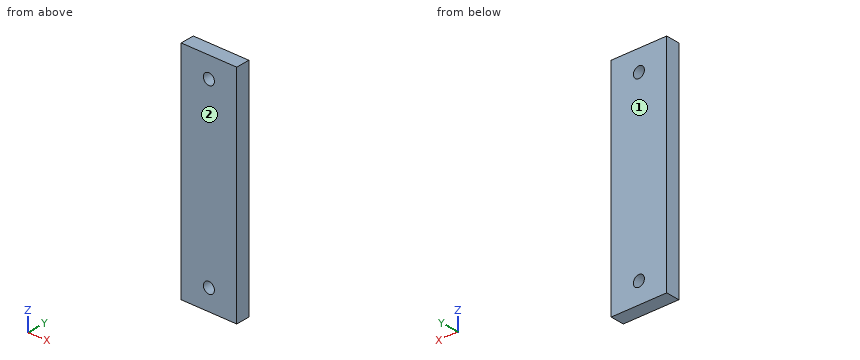
```python
from build123d import *

# Parameters (mm, degrees)
F0_W     = 50.8
F0_H     = 203.2
F1_DEPTH = 12.7
F2_D     = 10.0838
F2_DEPTH = 12.7
F2_TIP   = 3.0294791551


with BuildPart() as f1:
    # F0 (on Front) → F1 (new body)
    with BuildSketch(Plane.XZ):
        Rectangle(F0_W, F0_H)
    extrude(amount=F1_DEPTH)

    # F2
    with Locations(Plane(origin=(0, 0, 0), x_dir=(1, 0, 0), z_dir=(0, 1, 0))):
        with Locations((0, -82.55), (0, 82.55)):
            Hole(F2_D / 2, depth=F2_DEPTH)
            with Locations((0, 0, -(F2_DEPTH + F2_TIP / 2))):  # 118° drill point
                Cone(0, F2_D / 2, F2_TIP, mode=Mode.SUBTRACT)


solid = f1.part
```
Here's how the part is built. I have some questions about the finished solid (model axes, mm). Face numbers are marked on the shaded views. Give positions to 0.01 mm unless a question says otherwise; leave off trailing zeros. Order: outer loops, then holes, each group sorted by start corner. A loop starts at its lowest first (then second) coordinate and runs counter-clockwise, first axis right, second up. Notation, with made-up numbers: M 68,0 L 103,0 A22 ccw 103,15 Z; hole C 19,14 d5. An arc over 180 degrees is marked long. Use a Markdown table: item, result. Add a question column.
1. Suppose I cut it at B-B (x = 0). List the corners of the cut face in (y, z) for me.
2. I need wall thicknesses on probe 1 along Z at (x, y) = (0, -4.5); probe 2 along X at (y, z) = (-9, -82.55). Which ranges of each line are inside material? Lowest first, please. Write a range as from..to.
3. Suppose I cut it at C-C (y = -10.75). List the corners of the cut face in (x, z) for me.
4. Suppose I cut it at A-A (z = 82.55). List the corners of the cut face in (x, y) for me, and give its area (3 significant figures).
5. If we mould it in two halves opening along Y, with no side actions, what happens to the marked faces 1 and 2? For each: +Y half, -Y half, draft (parallel to the pull), parting line (faces both ways), or undercut.
Results list:
| question | item | result |
|---|---|---|
| 1 | outline | M -12.7,-101.6 L 0,-101.6 L 0,-87.59 L -12.7,-87.59 Z; M -12.7,-77.51 L 0,-77.51 L 0,77.51 L -12.7,77.51 Z; M -12.7,87.59 L 0,87.59 L 0,101.6 L -12.7,101.6 Z |
| 2 | probe 1 | z = -101.6..-87.59, -77.51..77.51, 87.59..101.6 |
| 2 | probe 2 | x = -25.4..-5.04, 5.04..25.4 |
| 3 | outline | M -25.4,-101.6 L 25.4,-101.6 L 25.4,101.6 L -25.4,101.6 Z; hole C 0,-82.55 d10.08; hole C 0,82.55 d10.08 |
| 4 | outline | M -25.4,-12.7 L -5.04,-12.7 L -5.04,0 L -25.4,0 Z; M 5.04,-12.7 L 25.4,-12.7 L 25.4,0 L 5.04,0 Z |
| 4 | area | 517 mm² |
| 5 | face 1 | +Y half |
| 5 | face 2 | -Y half |
